Build history of the part. All positions in model axes, mm. Face numbers are marked on the shaded views. A direction names the side the tool comes from. Give positions to 0.01 mm unless a question says otherwise; leave off trailing zeros. Order: outer loops, then holes, each group sorted by start corner. A loop starts at its lowest first (then second) coordinate and runs counter-clockwise, first axis right, second up. Notation, with made-up numbers: M 78.5,7.25 L 122.5,7.25 A17 ccw 122.5,17.25 Z; hole C 30.5,84 d8. An arc over 180 degrees is marked long. One line per item, written item: value. Start each with the question number.
from build123d import *

# Parameters (mm, degrees)
EXTRUDE_1_DEPTH                      = 0.65
CHAMFER_1_SIZE                       = 0.5
PATTERN_CIRCULAR_2_COUNT             = 4
CHAMFER_1_OF_PATTERN_CIRCULAR_2_SIZE = 0.5
FILLET_1_R                           = 0.1


with BuildPart() as part:
    # 스케치1 → 회전1 (revolve)
    with BuildSketch(Plane(origin=(0, 0, 0), x_dir=(1, 0, 0), z_dir=(0, 1, 0)), mode=Mode.PRIVATE) as revolve_1_sk:
        Polygon((0, 0), (1.5, 0.34993434), (2, 0.34993434), (2, -10), (1, -10), (1, -19.748270111), (0.7, -20), (0, -20), align=None)
    revolve(revolve_1_sk.sketch.rotate(Axis((0, 0, 0), (0, 0, 1)), 180), axis=Axis((0, 0, 0), (0, 0, 1)))

    # 스케치2 → 보스-돌출1 (add, symmetric)
    with BuildSketch(Plane(origin=(0, 0, 0), x_dir=(0, 0, -1), z_dir=(1, 0, 0))):
        Polygon((-10, 2.9), (1.575466057, 4.9), (7.420556651, 4.9), (7, 2.759707009), (0.34993434, 2), (0.34993434, 1.4), (-10, 1.4), align=None)
    extrude_1 = extrude(amount=EXTRUDE_1_DEPTH, both=True)

    # 모따기1
    chamfer_1_edges = [part.edges().sort_by_distance(p)[0] for p in [
        (0.65, 4.9, -4.498011354),
        (0.65, 3.9, 4.212266971),
        (-0.65, 4.9, -4.498011354),
        (-0.65, 3.9, 4.212266971),
    ]]
    chamfer(chamfer_1_edges, length=CHAMFER_1_SIZE)

    # 원형 패턴2: 보스-돌출1 ×4 about axis
    pattern_circular_2_axis = Axis((0, 0, 0), (0, 0, 1))
    for i in range(1, PATTERN_CIRCULAR_2_COUNT):
        add(extrude_1.rotate(pattern_circular_2_axis, i * 360 / PATTERN_CIRCULAR_2_COUNT))

    # 모따기1 of 원형 패턴2
    chamfer_1_of_pattern_circular_2_edges = [part.edges().sort_by_distance(p)[0] for p in [
        (-4.9, 0.65, -4.498011354),
        (-3.9, 0.65, 4.212266971),
        (-4.9, -0.65, -4.498011354),
        (-3.9, -0.65, 4.212266971),
        (-0.65, -4.9, -4.498011354),
        (-0.65, -3.9, 4.212266971),
        (0.65, -4.9, -4.498011354),
        (0.65, -3.9, 4.212266971),
        (4.9, -0.65, -4.498011354),
        (3.9, -0.65, 4.212266971),
        (4.9, 0.65, -4.498011354),
        (3.9, 0.65, 4.212266971),
    ]]
    chamfer(chamfer_1_of_pattern_circular_2_edges, length=CHAMFER_1_OF_PATTERN_CIRCULAR_2_SIZE)

    # 필렛1
    fillet_1_edges = [part.edges().sort_by_distance(p)[0] for p in [
        (0, -2, -0.34993434),
        (-1.414213562, 1.414213562, -0.34993434),
        (1.414213562, 1.414213562, -0.34993434),
        (0, 2, -0.34993434),
        (1.414213562, -1.414213562, -0.34993434),
        (2, 0, -0.34993434),
        (-1.414213562, -1.414213562, -0.34993434),
    ]]
    fillet(fillet_1_edges, radius=FILLET_1_R)

    # 스케치3 → 회전2 (revolve)
    with BuildSketch(Plane(origin=(0, 0, 0), x_dir=(0, 0, -1), z_dir=(1, 0, 0)), mode=Mode.PRIVATE) as revolve_2_sk:
        Polygon((-10, 2.9), (0, 0), (-10, 0), (-10, 2), (-11.378788521, 2), (-10.54680135, 2.9), align=None)
    revolve(revolve_2_sk.sketch.rotate(Axis((0, 0, 0), (0, 0, 1)), 90), axis=Axis((0, 0, 0), (0, 0, 1)))


solid = part.part
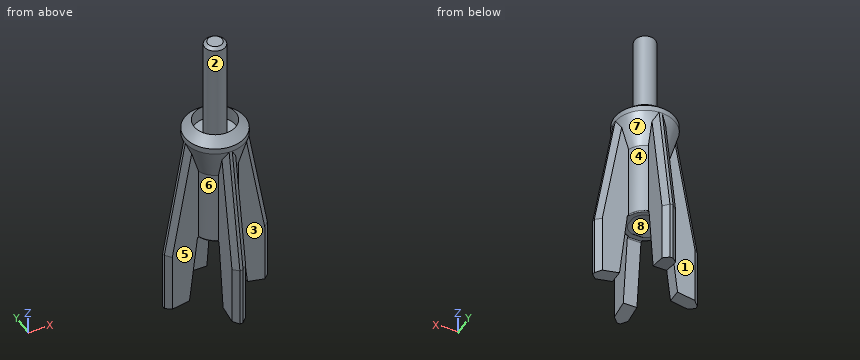
1) Slice it at A-A (z = -4.25). List the corners of the cut face in (x, y), plus the area to 3 significant figures.
2) Tool access for the marked faces 1, 2, 3 and 4: list every direction of +Z, -Z, +X, -X, +Y, -Y with a clear straight run to the whole face (end or side of a thin tool).
3) Drop flat-ended pins along their axis: P1, Ø2, axis at x = -0.5, z = 7.5, coming from the +Y side; P2, Ø1.1, axis at x = 0, y = 0, coming from the -Z side; P3, Ø1.3, axis at x = -3.5, z = 2, coming from the -Y side; P4, Ø2, axis at x = -2, y = -3.5, coming from the -Z side. Give the stop position or say it passes through.
4) Slice it at C-C (y = -4). List the corners of the cut face in (x, z), plus the area to 3 significant figures.
5) Slice it at B-B (z = 2.5). List the corners of the cut face in (x, y), plus the area to 3 significant figures.
6) Drill centre lines: line 1 (Y direction, x = 0, z = 10.6); line 2 (Y direction, x = 0, z = 11); line 3 (Z direction, x = -1.5, y = 0.5). Where is each one in solid material? Low to high.
7) Pull direction X, two halves, no side cores. Call the marked faces 5, 6, 7 and 8: pulls with the +X half, pulls with the -X half, needs draft (parallel to the pull), parting line crosses it, or undercut.
Results list:
1. outline: M -4.9,-0.15 L -4.4,-0.65 L -2.45,-0.65 L -2.45,0.65 L -4.4,0.65 L -4.9,0.15 Z; M -0.65,-4.4 L -0.15,-4.9 L 0.15,-4.9 L 0.65,-4.4 L 0.65,-2.45 L -0.65,-2.45 Z; M -0.65,2.45 L 0.65,2.45 L 0.65,4.4 L 0.15,4.9 L -0.15,4.9 L -0.65,4.4 Z; M 2.45,-0.65 L 4.4,-0.65 L 4.9,-0.15 L 4.9,0.15 L 4.4,0.65 L 2.45,0.65 Z
1. area: 11.8 mm²
2. face 1: -Z, -X, +Y
2. face 2: +Z
2. face 3: -Z, +X, -Y
2. face 4: -Z, +X, +Y
3. P1: stops at y = 3.49
3. P2: stops at z = -0.13
3. P3: stops at y = -0.65
3. P4: passes through
4. outline: M -0.65,-7.24 L 0.65,-7.24 L 0.65,0.7 L 0.15,3.63 L -0.15,3.63 L -0.65,0.7 Z
4. area: 12.7 mm²
5. outline: M -4.2,-0.15 L -3.69,-0.65 L -1.89,-0.65 A2 ccw -0.65,-1.89 L -0.65,-3.69 L -0.15,-4.2 L 0.15,-4.2 L 0.65,-3.69 L 0.65,-1.89 A2 ccw 1.89,-0.65 L 3.69,-0.65 L 4.2,-0.15 L 4.2,0.15 L 3.69,0.65 L 1.89,0.65 A2 ccw 0.65,1.89 L 0.65,3.69 L 0.15,4.2 L -0.15,4.2 L -0.65,3.69 L -0.65,1.89 A2 ccw -1.89,0.65 L -3.69,0.65 L -4.2,0.15 Z
5. area: 23.2 mm²
6. line 1: y = -2.84 to -2, -1 to 1, 2 to 2.84
6. line 2: y = -2.41 to -2, -1 to 1, 2 to 2.41
6. line 3: z = -0.35 to 10
7. face 5: needs draft
7. face 6: pulls with the -X half
7. face 7: pulls with the +X half
7. face 8: undercut
